from build123d import *

# Parameters (mm, degrees)
F1_DEPTH = 25.4


with BuildPart() as f1:
    # F0 (on Front) → F1 (new body)
    with BuildSketch(Plane.XZ):
        Polygon((-29.0627366167, 59.2265195809), (-26.5986134675, 51.6914901655), (4.8500286105, 49.9238849428), (4.8500286105, 70.576620616), (-19.5671229655, 68.4053798518), align=None)
        Polygon((31.3274671897, 72.9310678085), (4.8500286105, 49.9238849428), (42.4443297088, 47.8108562529), align=None)
        Polygon((4.8500286105, 70.576620616), (4.8500286105, 49.9238849428), (31.3274671897, 72.9310678085), align=None)
        Polygon((-36.2940447313, 52.2364324526), (-29.0627366167, 59.2265195809), (-31.7112803459, 67.3254877329), (-61.7150329053, 53.6652468145), align=None)
        Polygon((-31.7112803459, 67.3254877329), (-29.0627366167, 59.2265195809), (-19.5671229655, 68.4053798518), align=None)
        Polygon((-51.8806073309, 37.1698042746), (-36.2940447313, 52.2364324526), (-61.7150329053, 53.6652468145), align=None)
        Polygon((-65.600423, 7.4018295103), (-40.8824269365, 18.7223767795), (-51.8806073309, 37.1698042746), (-61.7150329053, 53.6652468145), (-70.7405507565, -49.0305200219), (-68.4894029233, -24.315655452), align=None)
        Polygon((71.4723467827, 47.8108562529), (42.4443297088, 47.8108562529), (46.4224250242, 41.3202796856), (69.8888571857, 42.2007769877), align=None)
        Polygon((56.1034718341, 75.1342187818), (42.4443297088, 47.8108562529), (71.4723467827, 47.8108562529), (71.4723467827, 50.058685971), align=None)
        Polygon((31.3274671897, 72.9310678085), (42.4443297088, 47.8108562529), (56.1034718341, 75.1342187818), align=None)
        Polygon((69.8888571857, 42.2007769877), (46.4224250242, 41.3202796856), (49.9897200646, 35.4999561987), align=None)
        Polygon((15.9801721379, -35.6691343344), (5.2863502547, -45.8093752593), (14.6359754726, -74.3995457888), (38.7853346765, -38.0608700216), align=None)
        Polygon((14.6359754726, -74.3995457888), (5.2863502547, -45.8093752593), (0.3700881163, -50.4711400688), align=None)
        Polygon((-57.13157103, -37.3866297692), (-68.4894029233, -24.315655452), (-70.7405507565, -49.0305200219), align=None)
        Polygon((-57.13157103, -37.3866297692), (-70.7405507565, -49.0305200219), (-50.6175059134, -44.8832346352), align=None)
        Polygon((-50.6175059134, -44.8832346352), (-70.7405507565, -49.0305200219), (-38.7552418775, -58.5347263998), align=None)
        Polygon((69.8888571857, 42.2007769877), (49.9897200646, 35.4999561987), (60.9832331538, 17.5631716847), (62.9346966743, 17.5631716847), align=None)
        Polygon((-17.4304527242, -64.8712353842), (14.6359754726, -74.3995457888), (0.3700881163, -50.4711400688), (-21.9214353892, -55.0653409168), align=None)
        Polygon((38.7853346765, -38.0608700216), (14.6359754726, -74.3995457888), (54.5582934135, -74.3995457888), align=None)
        Polygon((-21.9214353892, -55.0653409168), (-28.6575145446, -40.3573613388), (-50.6175059134, -44.8832346352), (-38.7552418775, -58.5347263998), align=None)
        Polygon((60.9832331538, 17.5631716847), (38.7853346765, -38.0608700216), (54.5582934135, -74.3995457888), (62.9346966743, 17.5631716847), align=None)
        Polygon((-21.9214353892, -55.0653409168), (-38.7552418775, -58.5347263998), (-17.4304527242, -64.8712353842), align=None)
    extrude(amount=F1_DEPTH)


solid = f1.part
The listing builds one solid part. Answer for the finished solid, in the listing's coordinates (mm). A direction names the side the tool comes from. Round coordinates to 2 decimals unless told otherwise and drop trailing zeros. Write each loop counter-clockwise with the first axis right and the second up, starting at its lowest first coordinate (ties: lowest second). Pieces come first, ordered by that corner, then holes. Notation, with made-up numbers: (66.5, 48) - (119.5, 48) arc R22 cw to (119.5, 64) - close; hole circle Ø5 at (11.25, 51.25). An arc over 180 degrees is marked (long way). Use a Markdown table: item, result. Add a question column.
1. Flat-ended cylindrical pins translate along their axes: P1, Ø1, axis at x = -32.5, y = -22, coming from the -Z side; P2, Ø10, axis at y = -11.5, z = 33.5, coming from the +X side; P3, Ø1.5, axis at y = -17.5, z = -23, coming from the +X side. Find the tip coordinate at first contact, or state that the pin passes through.
2. The part is cut by section D-D (z = 64.5). Write down the section's boundary in (x, y).
3. A tool of negligible diameter and unlimited length cuts with its end or side. For faces 1 (the face through (63.895, -12.522, 62.421)), 2 (the face through (-10.62, -12.522, -52.736)), from which of +Z, -Z, +X, -X, +Y, -Y can it reach the whole face along a straight path? Write none if from no direction.
4. The part is cut by section C-C (x = -15). Write down the section's boundary in (y, z), and give its area (3 significant figures).
5. The part is cut by section B-B (z = -27). Write down the section's boundary in (x, y).
6. The part is cut by section A-A (y = -15.75). Write down the section's boundary in (x, z).
7. Consider line 1 (X direction, y = -19.5, z = 0); line 2 (Z direction, x = -2.5, y = -13); line 3 (X direction, y = -20.25, z = 55.5). Determine where each line is inside the solid, lowest interval first.
Reported:
| question | item | result |
|---|---|---|
| 1 | P1 | z = -60.54 |
| 1 | P2 | x = 68.84 |
| 1 | P3 | x = 59.31 |
| 2 | outline | (-37.92, -25.4) - (62.62, -25.4) - (62.62, 0) - (-37.92, 0) - close |
| 3 | face 1 | +Z, +X, +Y, -Y |
| 3 | face 2 | +Y, -Y |
| 4 | outline | (-25.4, -65.59) - (0, -65.59) - (0, -53.64) - (-25.4, -53.64) - close; (-25.4, 51.04) - (0, 51.04) - (0, 68.81) - (-25.4, 68.81) - close |
| 4 | area | 755 mm^2 |
| 5 | outline | (-68.8, -25.4) - (-66.16, -25.4) - (-66.16, 0) - (-68.8, 0) - close; (43.2, -25.4) - (58.88, -25.4) - (58.88, 0) - (43.2, 0) - close |
| 6 | outline | (-70.74, -49.03) - (14.64, -74.4) - (54.56, -74.4) - (62.93, 17.56) - (71.47, 47.81) - (71.47, 50.06) - (56.1, 75.13) - (-31.71, 67.33) - (-61.72, 53.67) - close; hole (-68.49, -24.32) - (-50.62, -44.88) - (-28.66, -40.36) - (-21.92, -55.07) - (0.37, -50.47) - (15.98, -35.67) - (38.79, -38.06) - (60.98, 17.56) - (42.44, 47.81) - (-26.6, 51.69) - (-29.06, 59.23) - (-51.88, 37.17) - (-40.88, 18.72) - (-65.6, 7.4) - close |
| 7 | line 1 | -66.43 to -66.27, 53.97 to 61.33 |
| 7 | line 2 | -69.31 to -51.06, 50.34 to 69.92 |
| 7 | line 3 | -57.69 to -32.92, -27.84 to 68.14 |
